from build123d import *

# Parameters (mm, degrees)
CROQUIS1_W              = 62
CROQUIS1_H              = 62
SALIENTE_EXTRUIR1_DEPTH = 6.5
REDONDEO1_R             = 10
REDONDEO2_R             = 10
VACIADO1_T              = -2.5
SALIENTE_EXTRUIR2_DEPTH = 5
CROQUIS6_R              = 12.25
CORTAR_EXTRUIR4_DEPTH   = 4
CROQUIS8_R              = 10.5
CORTAR_EXTRUIR7_DEPTH   = 70.535961919
CROQUIS9_R              = 1.65
CORTAR_EXTRUIR8_DEPTH   = 70.622194737
CROQUIS10_R             = 3.325
CORTAR_EXTRUIR9_DEPTH   = 3
SALIENTE_EXTRUIR3_START = 1.5
CROQUIS11_R             = 3.910048181
CROQUIS11_R_2           = 1.65
CROQUIS11_R_3           = 3.794929079
CROQUIS11_R_4           = 3.596875763
SALIENTE_EXTRUIR3_DEPTH = 1.5
REDONDEO3_R             = 2
CHAFL_N1_SIZE           = 1
CHAFL_N2_SIZE           = 2
CROQUIS12_R             = 5.75
CORTAR_EXTRUIR10_DEPTH  = 4
CHAFL_N3_SIZE           = 1
CORTAR_EXTRUIR11_DEPTH  = 3
CHAFL_N4_SIZE           = 2


with BuildPart() as part:
    # Croquis1 → Saliente-Extruir1 (new body)
    with BuildSketch(Plane(origin=(0, 0, 0), x_dir=(1, 0, 0), z_dir=(0, 1, 0))):
        with Locations((31, 0)):
            Rectangle(CROQUIS1_W, CROQUIS1_H)
    extrude(amount=SALIENTE_EXTRUIR1_DEPTH)

    # Redondeo1
    redondeo1_edges = [part.edges().sort_by_distance(p)[0] for p in [
        (62, 3.25, -31),
        (62, 3.25, 31),
    ]]
    fillet(redondeo1_edges, radius=REDONDEO1_R)

    # Redondeo2
    redondeo2_edges = [part.edges().sort_by_distance(p)[0] for p in [
        (0, 3.25, -31),
        (0, 3.25, 31),
    ]]
    fillet(redondeo2_edges, radius=REDONDEO2_R)

    # Vaciado1
    vaciado1_openings = [part.faces().sort_by_distance(p)[0] for p in [
        (31, 6.5, 0),
        (31, 0, 0),
    ]]
    offset(amount=VACIADO1_T, openings=vaciado1_openings, kind=Kind.INTERSECTION)

    # Croquis4 → Saliente-Extruir2 (add)
    with BuildSketch(Plane.XZ.offset(-6.5)):
        with BuildLine():
            Line((7.085748882, 28.5), (54.5, 28.5))
            ThreePointArc((54.5, 28.5), (58.035533906, 27.035533906), (59.5, 23.5))
            Line((59.5, 23.5), (59.5, -23.5))
            ThreePointArc((59.5, -23.5), (58.035533906, -27.035533906), (54.5, -28.5))
            Line((54.5, -28.5), (7.085748882, -28.5))
            ThreePointArc((7.085748882, -28.5), (3.550214976, -27.035533906), (2.085748882, -23.5))
            Line((2.085748882, -23.5), (2.085748882, 23.5))
            ThreePointArc((2.085748882, 23.5), (3.550214976, 27.035533906), (7.085748882, 28.5))
        make_face()
    extrude(amount=SALIENTE_EXTRUIR2_DEPTH)

    # Croquis6 → Cortar-Extruir4 (cut)
    with BuildSketch(Plane(origin=(0, 1.5, 0), x_dir=(-1, 0, 0), z_dir=(0, -1, 0))):
        with Locations(Location((-16.5, 0, 0), (0, 0, 90))):
            Circle(CROQUIS6_R)
    extrude(amount=-CORTAR_EXTRUIR4_DEPTH, mode=Mode.SUBTRACT)

    # Croquis8 → Cortar-Extruir7 (cut, through all)
    with BuildSketch(Plane.XZ.offset(-5.5)):
        with Locations(Location((16.5, 0, 0), (0, 0, 270))):
            Circle(CROQUIS8_R)
    extrude(amount=-CORTAR_EXTRUIR7_DEPTH, mode=Mode.SUBTRACT)

    # Croquis9 → Cortar-Extruir8 (cut, through all)
    with BuildSketch(Plane.XZ):
        with Locations(Location((6, 25, 0), (0, 0, 270))):
            Circle(CROQUIS9_R)
        with Locations(Location((56, 25, 0), (0, 0, 270))):
            Circle(CROQUIS9_R)
        with Locations(Location((56, -25, 0), (0, 0, 270))):
            Circle(CROQUIS9_R)
        with Locations(Location((6, -25, 0), (0, 0, 270))):
            Circle(CROQUIS9_R)
    extrude(amount=-CORTAR_EXTRUIR8_DEPTH, mode=Mode.SUBTRACT)

    # Croquis10 → Cortar-Extruir9 (cut)
    with BuildSketch(Plane(origin=(0, 6.5, 0), x_dir=(1, 0, 0), z_dir=(0, 1, 0))):
        with Locations(Location((6, 25, 0), (0, 0, 270))):
            Circle(CROQUIS10_R)
        with Locations(Location((6, -25, 0), (0, 0, 270))):
            Circle(CROQUIS10_R)
        with Locations(Location((56, -25, 0), (0, 0, 270))):
            Circle(CROQUIS10_R)
        with Locations(Location((56, 25, 0), (0, 0, 270))):
            Circle(CROQUIS10_R)
    extrude(amount=-CORTAR_EXTRUIR9_DEPTH, mode=Mode.SUBTRACT)

    # Croquis11 → Saliente-Extruir3 (add)
    # profile 1 of 4: a face of its own
    with BuildSketch(Plane.XZ.offset(-1.5).offset(SALIENTE_EXTRUIR3_START)):
        with Locations((6, 25)):
            Circle(CROQUIS11_R)
        with Locations(Location((6, 25, 0), (0, 0, 270))):
            Circle(CROQUIS11_R_2, mode=Mode.SUBTRACT)
    # profile 2 of 4: a face of its own
    with BuildSketch(Plane.XZ.offset(-1.5).offset(SALIENTE_EXTRUIR3_START)):
        with Locations((6, -25)):
            Circle(CROQUIS11_R_3)
        with Locations(Location((6, -25, 0), (0, 0, 270))):
            Circle(CROQUIS11_R_2, mode=Mode.SUBTRACT)
    # profile 3 of 4: a face of its own
    with BuildSketch(Plane.XZ.offset(-1.5).offset(SALIENTE_EXTRUIR3_START)):
        with Locations((56, -25)):
            Circle(CROQUIS11_R_4)
        with Locations(Location((56, -25, 0), (0, 0, 270))):
            Circle(CROQUIS11_R_2, mode=Mode.SUBTRACT)
    # profile 4 of 4: a face of its own
    with BuildSketch(Plane.XZ.offset(-1.5).offset(SALIENTE_EXTRUIR3_START)):
        with Locations((56, 25)):
            Circle(CROQUIS11_R_4)
        with Locations(Location((56, 25, 0), (0, 0, 270))):
            Circle(CROQUIS11_R_2, mode=Mode.SUBTRACT)
    extrude(amount=-SALIENTE_EXTRUIR3_DEPTH)

    # Redondeo3
    redondeo3_edges = [part.edges().sort_by_distance(p)[0] for p in [
        (54.263904065, 0.75, 28.150156529),
        (59.150156529, 0.75, 23.263904065),
        (59.150156529, 0.75, -23.263904065),
        (54.263904065, 0.75, -28.150156529),
        (7.996337674, 0.75, -28.227401835),
        (2.772598165, 0.75, -23.003662326),
        (2.732409322, 0.75, 22.852599726),
        (8.147400274, 0.75, 28.267590678),
    ]]
    fillet(redondeo3_edges, radius=REDONDEO3_R)

    # Chaflán1
    chafl_n1_edges = [part.edges().sort_by_distance(p)[0] for p in [
        (16.5, 1.5, 12.25),
    ]]
    chamfer(chafl_n1_edges, length=CHAFL_N1_SIZE)

    # Chaflán2
    # the kernel refuses this chamfer: 2 mm, written as the material it takes off along each edge
    with BuildSketch(Plane(origin=(10, 6.5, -31), x_dir=(0, -0.9996219169112968, -0.027495876610585623), z_dir=(1, 0, 0)), Plane(origin=(62, 6.5, -21), x_dir=(0.027495876610585623, -0.9996219169112968, 0), z_dir=(0, 0, 1)), Plane(origin=(52, 6.5, 31), x_dir=(0, -0.9996219169112968, 0.027495876610585623), z_dir=(-1, 0, 0)), Plane(origin=(0, 6.5, 21), x_dir=(-0.027495876610586365, -0.9996219169112968, 0), z_dir=(0, 0, -1))) as chafl_n2_piece_1:
        Polygon((CHAFL_N2_SIZE * 0.999621916911, -CHAFL_N2_SIZE * 0.0274958766106), (-CHAFL_N2_SIZE * 0.0274958766106, -CHAFL_N2_SIZE * 0.999621916911), (0, 0), align=None)
    extrude(amount=42, mode=Mode.SUBTRACT)
    with BuildSketch(Plane(origin=(52, 6.5, 21), x_dir=(1, 0, 0), z_dir=(0, 0, -1))) as chafl_n2_piece_2:
        Polygon((10, CHAFL_N2_SIZE), (10 - CHAFL_N2_SIZE, 0), (10, 0), align=None)
    revolve(axis=Axis((52, 6.5, 21), (0, -1, 0)), revolution_arc=90, mode=Mode.SUBTRACT)
    with BuildSketch(Plane(origin=(52, 6.5, -21), x_dir=(0, 0, -1), z_dir=(-1, 0, 0))) as chafl_n2_piece_3:
        Polygon((10, CHAFL_N2_SIZE), (10 - CHAFL_N2_SIZE, 0), (10, 0), align=None)
    revolve(axis=Axis((52, 6.5, -21), (0, -1, 0)), revolution_arc=90, mode=Mode.SUBTRACT)
    with BuildSketch(Plane(origin=(10, 6.5, -21), x_dir=(0, 0, -1), z_dir=(1, 0, 0))) as chafl_n2_piece_4:
        Polygon((10, -CHAFL_N2_SIZE), (10 - CHAFL_N2_SIZE, 0), (10, 0), align=None)
    revolve(axis=Axis((10, 6.5, -21), (0, 1, 0)), revolution_arc=90, mode=Mode.SUBTRACT)
    with BuildSketch(Plane(origin=(10, 6.5, 21), x_dir=(-1, 0, 0), z_dir=(0, 0, -1))) as chafl_n2_piece_5:
        Polygon((10, -CHAFL_N2_SIZE), (10 - CHAFL_N2_SIZE, 0), (10, 0), align=None)
    revolve(axis=Axis((10, 6.5, 21), (0, 1, 0)), revolution_arc=90, mode=Mode.SUBTRACT)

    # Croquis12 → Cortar-Extruir10 (cut)
    with BuildSketch(Plane.XZ.offset(-1.5)):
        with Locations(Location((44, 0, 0), (0, 0, 270))):
            Circle(CROQUIS12_R)
    extrude(amount=-CORTAR_EXTRUIR10_DEPTH, mode=Mode.SUBTRACT)

    # Chaflán3
    chafl_n3_edges = [part.edges().sort_by_distance(p)[0] for p in [
        (44, 1.5, 5.75),
    ]]
    chamfer(chafl_n3_edges, length=CHAFL_N3_SIZE)

    # Croquis14 → Cortar-Extruir11 (cut)
    with BuildSketch(Plane.XZ.offset(-1.5)):
        with BuildLine():
            Line((20.919533653, 24.89123626), (43.446250752, 24.89123626))
            ThreePointArc((43.446250752, 24.89123626), (44.211617617, 24.738995325), (44.860464315, 24.305449822))
            Line((44.860464315, 24.305449822), (51.391720064, 17.774194073))
            ThreePointArc((51.391720064, 17.774194073), (51.825265567, 17.125347375), (51.977506502, 16.35998051))
            Line((51.977506502, 16.35998051), (51.977506502, 13.625253628))
            ThreePointArc((51.977506502, 13.625253628), (51.391720064, 12.211040066), (49.977506502, 11.625253628))
            Line((49.977506502, 11.625253628), (39.986196606, 11.625253628))
            ThreePointArc((39.986196606, 11.625253628), (39.678099546, 11.649127063), (39.37735782, 11.720177427))
            Line((39.37735782, 11.720177427), (20.310694867, 17.81364703))
            ThreePointArc((20.310694867, 17.81364703), (19.304343638, 18.539248258), (18.919533653, 19.718723232))
            Line((18.919533653, 19.718723232), (18.919533653, 22.89123626))
            ThreePointArc((18.919533653, 22.89123626), (19.505320091, 24.305449822), (20.919533653, 24.89123626))
        make_face()
        with BuildLine():
            Line((18.919533653, -19.718723232), (18.919533653, -22.89123626))
            ThreePointArc((18.919533653, -22.89123626), (19.505320091, -24.305449822), (20.919533653, -24.89123626))
            Line((20.919533653, -24.89123626), (43.446250752, -24.89123626))
            ThreePointArc((43.446250752, -24.89123626), (44.211617617, -24.738995325), (44.860464315, -24.305449822))
            Line((44.860464315, -24.305449822), (51.391720064, -17.774194073))
            ThreePointArc((51.391720064, -17.774194073), (51.825265567, -17.125347375), (51.977506502, -16.35998051))
            Line((51.977506502, -16.35998051), (51.977506502, -13.625253628))
            ThreePointArc((51.977506502, -13.625253628), (51.391720064, -12.211040066), (49.977506502, -11.625253628))
            Line((49.977506502, -11.625253628), (39.986196606, -11.625253628))
            ThreePointArc((39.986196606, -11.625253628), (39.678099546, -11.649127063), (39.37735782, -11.720177427))
            Line((39.37735782, -11.720177427), (20.310694867, -17.81364703))
            ThreePointArc((20.310694867, -17.81364703), (19.304343638, -18.539248258), (18.919533653, -19.718723232))
        make_face()
    extrude(amount=-CORTAR_EXTRUIR11_DEPTH, mode=Mode.SUBTRACT)

    # Chaflán4
    chafl_n4_edges = [part.edges().sort_by_distance(p)[0] for p in [
        (39.678099546, 1.5, 11.649127063),
        (44.981851554, 1.5, 11.625253628),
        (51.391720064, 1.5, 12.211040066),
        (51.977506502, 1.5, 14.992617069),
        (51.825265567, 1.5, 17.125347375),
        (48.12609219, 1.5, 21.039821948),
        (44.211617617, 1.5, 24.738995325),
        (32.182892203, 1.5, 24.89123626),
        (19.505320091, 1.5, 24.305449822),
        (18.919533653, 1.5, 21.304979746),
        (19.304343638, 1.5, 18.539248258),
        (29.844026344, 1.5, 14.766912229),
        (19.505320091, 1.5, -24.305449822),
        (32.182892203, 1.5, -24.89123626),
        (44.211617617, 1.5, -24.738995325),
        (48.12609219, 1.5, -21.039821948),
        (51.825265567, 1.5, -17.125347375),
        (51.977506502, 1.5, -14.992617069),
        (51.391720064, 1.5, -12.211040066),
        (44.981851554, 1.5, -11.625253628),
        (39.678099546, 1.5, -11.649127063),
        (29.844026344, 1.5, -14.766912229),
        (19.304343638, 1.5, -18.539248258),
        (18.919533653, 1.5, -21.304979746),
    ]]
    chamfer(chafl_n4_edges, length=CHAFL_N4_SIZE)


solid = part.part
Could you check a few things on this model? Use its own coordinates, in mm. A direction names the side the tool comes from. Round coordinates to 2 decimals unless told otherwise and drop trailing zeros. Write each loop counter-clockwise with the first axis right and the second up, starting at its lowest first coordinate (ties: lowest second). Pieces come first, ordered by that corner, then holes. Notation, with made-up numbers: (36, -34) -> (69, -34) arc R22 ccw to (69, -1) -> close; hole circle Ø4 at (58.5, 14). An arc over 180 degrees is marked (long way). Use a Markdown table: item, result.
1. For pin 1 Ø1.5 at (x, y) = (7, 1) entering from -Z; pin 2 Ø6.5 at (x, z) = (43.5, 16.5) entering from -Y; pin 3 Ø6 at (x, z) = (43.5, 2) entering from -Y, each with a flat end and sliding along its axis, tell me the tip position at first contact or that it passes through.
Answer key:
| item | result |
|---|---|
| pin 1 | stops at z = -30.74 |
| pin 2 | stops at y = 4.5 |
| pin 3 | stops at y = 5.5 |
2. Please list where these lines run through material, in increasing order: probe 1 along X at (y, z) = (4.4, 25) (3 decimals); probe 2 along X at (y, z) = (5, -2.5); probe 3 along Z at (x, y) = (46.5, 4.25).
Answer key:
| item | result |
|---|---|
| probe 1 | x = 0.835 to 2.675, 9.325 to 52.675, 59.325 to 61.165 |
| probe 2 | x = 0.5 to 4.51, 28.49 to 38.82, 49.18 to 61.5 |
| probe 3 | z = -31 to -22.67, -11.63 to -5.18, 5.18 to 11.63, 22.67 to 31 |
3. Which directions (+Z, -Z, +X, -X, +Y, -Y) give clear straight access to the entire face, cutting with the end or side of a thin tool? Please do faces 1 (the face through (36, 4.5, 18)), 2 (the face through (6.07, 1.73, -23.35)), 3 (the face through (53.98, 5.02, 22.36)).
Answer key:
| item | result |
|---|---|
| face 1 | -Y |
| face 2 | +Y, -Y |
| face 3 | +Y |
4. If we section it at A-A (x = 33): List the corners of the cut face in (y, z) for me.
Answer key:
| item | result |
|---|---|
| outline | (0, -31) -> (4.5, -31) -> (6.5, -29) -> (6.5, 29) -> (4.5, 31) -> (0, 31) -> (0, 28.5) -> (1.5, 28.5) -> (1.5, 26.89) -> (3.5, 24.89) -> (4.5, 24.89) -> (4.5, 13.76) -> (3.5, 13.76) -> (1.5, 11.66) -> (1.5, -11.66) -> (3.5, -13.76) -> (4.5, -13.76) -> (4.5, -24.89) -> (3.5, -24.89) -> (1.5, -26.89) -> (1.5, -28.5) -> (0, -28.5) -> close |
5. We'd pull the mould along X, two halves only. Please class faces 4 (the face through (31.3, 5.5, 30)), 5 (the face through (4.541, 3.979, 2.656)): +X half, -X half, draft (parallel to the pull), parting line (faces both ways), or undercut.
Answer key:
| item | result |
|---|---|
| face 4 | draft |
| face 5 | undercut |
